Read the model definition and answer for the solid it produces. Units are mm, in the model's axes. Coordinates: 2 decimals unless noted, no trailing zeros. Order: outer loops, then holes, each group sorted by start corner. A loop starts at its lowest first (then second) coordinate and runs counter-clockwise, first axis right, second up.
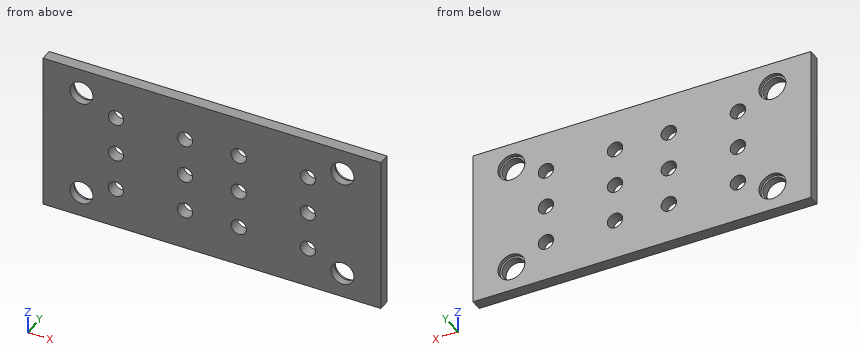
from build123d import *

# Parameters (mm, degrees)
SKETCH1_W           = 880
SKETCH1_H           = 410
BOSS_EXTRUDE1_DEPTH = 30
SKETCH2_R           = 30
CUT_EXTRUDE1_DEPTH  = 225
SKETCH3_R           = 35
CUT_EXTRUDE2_DEPTH  = 10
SKETCH4_R           = 20
CUT_EXTRUDE3_DEPTH  = 154


with BuildPart() as part:
    # Sketch1 → Boss-Extrude1 (new body)
    with BuildSketch(Plane(origin=(0, 0, 0), x_dir=(1, 0, 0), z_dir=(0, 1, 0))):
        Rectangle(SKETCH1_W, SKETCH1_H)
    extrude(amount=BOSS_EXTRUDE1_DEPTH)

    # Sketch2 → Cut-Extrude1 (cut)
    with BuildSketch(Plane(origin=(0, 30, 0), x_dir=(1, 0, 0), z_dir=(0, 1, 0))):
        with Locations(Location((-340, 140, 0), (0, 0, 270))):
            Circle(SKETCH2_R)
        with Locations(Location((340, 140, 0), (0, 0, 270))):
            Circle(SKETCH2_R)
        with Locations(Location((340, -140, 0), (0, 0, 270))):
            Circle(SKETCH2_R)
        with Locations(Location((-340, -140, 0), (0, 0, 270))):
            Circle(SKETCH2_R)
    extrude(amount=-CUT_EXTRUDE1_DEPTH, mode=Mode.SUBTRACT)

    # Sketch3 → Cut-Extrude2 (cut)
    with BuildSketch(Plane(origin=(0, 30, 0), x_dir=(1, 0, 0), z_dir=(0, 1, 0))):
        with Locations(Location((-340, 140, 0), (0, 0, 270))):
            Circle(SKETCH3_R)
        with Locations((-340, -540)):
            Circle(SKETCH3_R)
        with Locations((-340, -820)):
            Circle(SKETCH3_R)
        with Locations(Location((-340, -140, 0), (0, 0, 270))):
            Circle(SKETCH3_R)
        with Locations(Location((340, 140, 0), (0, 0, 270))):
            Circle(SKETCH3_R)
        with Locations(Location((340, -140, 0), (0, 0, 270))):
            Circle(SKETCH3_R)
    extrude(amount=-CUT_EXTRUDE2_DEPTH, mode=Mode.SUBTRACT)

    # Sketch4 → Cut-Extrude3 (cut)
    with BuildSketch(Plane(origin=(0, 30, 0), x_dir=(1, 0, 0), z_dir=(0, 1, 0))):
        with Locations(Location((-250, 0, 0), (0, 0, 270))):
            Circle(SKETCH4_R)
        with Locations(Location((-70, 0, 0), (0, 0, 270))):
            Circle(SKETCH4_R)
        with Locations(Location((-250, 100, 0), (0, 0, 270))):
            Circle(SKETCH4_R)
        with Locations(Location((-250, -100, 0), (0, 0, 270))):
            Circle(SKETCH4_R)
        with Locations(Location((-70, 100, 0), (0, 0, 270))):
            Circle(SKETCH4_R)
        with Locations(Location((-70, -100, 0), (0, 0, 270))):
            Circle(SKETCH4_R)
        with Locations(Location((70, -100, 0), (0, 0, 270))):
            Circle(SKETCH4_R)
        with Locations(Location((70, 100, 0), (0, 0, 270))):
            Circle(SKETCH4_R)
        with Locations(Location((250, -100, 0), (0, 0, 270))):
            Circle(SKETCH4_R)
        with Locations(Location((250, 100, 0), (0, 0, 270))):
            Circle(SKETCH4_R)
        with Locations(Location((70, 0, 0), (0, 0, 270))):
            Circle(SKETCH4_R)
        with Locations(Location((250, 0, 0), (0, 0, 270))):
            Circle(SKETCH4_R)
    extrude(amount=-CUT_EXTRUDE3_DEPTH, mode=Mode.SUBTRACT)


solid = part.part
Q1. The part is cut by section A-A, the plane z = -140. Determine the outline of the cut face in (x, y), then the cut area to 3 significant figures.
Q2. Straight lines are drawn through the part: L1, parallel to X at y = 10.25, z = 0; L2, parallel to Z at x = -249.5, y = 27.5; L3, parallel to Z at x = -349, y = 5. For each, find the intervals that lie inside material, in ascending order.
Q3. The part is cut by section D-D, the plane y = 10. State how many separate pieces and enclosed holes the cut face has, then the cut area to 3 significant figures.
Q4. The part is cut by section B-B, the plane x = 70. Determine the outline of the cut face in (y, z), then the cut area to 3 significant figures.
Q5. The part is cut by section C-C, the plane z = 0. Determine the outline of the cut face in (x, y).
Computed values:
1. outline: (-440, 0) - (-370, 0) - (-370, 20) - (-375, 20) - (-375, 30) - (-440, 30) - close; (-310, 0) - (310, 0) - (310, 20) - (305, 20) - (305, 30) - (-305, 30) - (-305, 20) - (-310, 20) - close; (370, 0) - (440, 0) - (440, 30) - (375, 30) - (375, 20) - (370, 20) - close
1. area: 22,600 mm2
2. L1: x = -440 to -270, -230 to -90, -50 to 50, 90 to 230, 270 to 440
2. L2: z = -205 to -119.99, -80.01 to -19.99, 19.99 to 80.01, 119.99 to 205
2. L3: z = -205 to -168.62, -111.38 to 111.38, 168.62 to 205
3. separate pieces: 1
3. enclosed holes: 16
3. area: 334,000 mm2
4. outline: (0, -205) - (30, -205) - (30, -120) - (0, -120) - close; (0, -80) - (30, -80) - (30, -20) - (0, -20) - close; (0, 20) - (30, 20) - (30, 80) - (0, 80) - close; (0, 120) - (30, 120) - (30, 205) - (0, 205) - close
4. area: 8,700 mm2
5. outline: (-440, 0) - (-270, 0) - (-270, 30) - (-440, 30) - close; (-230, 0) - (-90, 0) - (-90, 30) - (-230, 30) - close; (-50, 0) - (50, 0) - (50, 30) - (-50, 30) - close; (90, 0) - (230, 0) - (230, 30) - (90, 30) - close; (270, 0) - (440, 0) - (440, 30) - (270, 30) - close
